from build123d import *

# Parameters (mm, degrees)
F1_DEPTH = 152.4


# Not quite as in the source:
# - ends of sketch curves that miss each other by under 0.0002 mm in the source are joined


with BuildPart() as f1:
    # F0 (on Front) → F1 (new body)
    with BuildSketch(Plane.XZ):
        with BuildLine():
            ThreePointArc((-3.173984, 31.7550292), (-5.034153519, 36.245875681), (-9.525, 38.1060452))
            Line((-9.525, 38.1060452), (-9.525, -38.1060452))
            ThreePointArc((-9.525, -38.1060452), (-5.034153519, -36.245875681), (-3.173984, -31.7550292))
            ThreePointArc((-3.173984, -31.7550292), (1.3873070975, -29.8232975079), (3.1738358164, -25.2031917651))
            ThreePointArc((3.1738358164, -25.2031917651), (6.6091861803, -22.9435143548), (7.940294, -19.0530226))
            ThreePointArc((7.940294, -19.0530226), (7.2093686546, -16.094985199), (5.1848340025, -13.817816657))
            ThreePointArc((5.1848340025, -13.817816657), (9.5132844595, -8.141e-06), (5.1848116567, 13.8177933751))
            ThreePointArc((5.1848116567, 13.8177933751), (7.2093653059, 16.0949788365), (7.940294, 19.0530226))
            ThreePointArc((7.940294, 19.0530226), (6.6091861803, 22.9435143548), (3.1738358164, 25.2031917651))
            ThreePointArc((3.1738358164, 25.2031917651), (1.3873169736, 29.8232821056), (-3.173984, 31.7550292))
        make_face()
    extrude(amount=F1_DEPTH)


solid = f1.part
Could you check a few things on this model? Use its own coordinates, in mm. A direction names the side the tool comes from. Give positions to 0.01 mm unless a question says otherwise; leave off trailing zeros. Write each loop counter-clockwise with the first axis right and the second up, starting at its lowest first coordinate (ties: lowest second). Pieces come first, ordered by that corner, then holes. Notation, with made-up numbers: (-14, 12.5) -> (14, 12.5) arc R26 ccw to (14, 32.5) -> close; hole circle Ø2 at (-34, 13). An arc over 180 degrees is marked (long way). Answer as a JSON object with one key per item and string values.
Q1. Which directions (+Z, -Z, +X, -X, +Y, -Y) give clear straight access to the entire face, cutting with the end or side of a thin tool? Please do faces 4 (the cylindrical face through (7.19, -75.13, 16.06)), 5 (the cylindrical face through (-4.99, -75.13, 36.2)).
Taken from the geometry:
{"face 4": "+X, +Y, -Y", "face 5": "+Z, +X, +Y, -Y"}
Q2. Suppose I cut it at C-C on z = 5. Write out the boundary of the cut face in (x, y) (3 decimals), then the cut area to 3 significant figures.
Taken from the geometry:
{"outline": "(-9.525, -152.4) -> (8.992, -152.4) -> (8.992, 0) -> (-9.525, 0) -> close", "area": "2,820 mm²"}
Q3. Suppose I cut it at B-B on x = -1. Write out the boundary of the cut face in (y, z), then the cut area to 3 significant figures.
Taken from the geometry:
{"outline": "(-152.4, -31.37) -> (0, -31.37) -> (0, 31.37) -> (-152.4, 31.37) -> close", "area": "9,560 mm²"}
Q4. Will these pins go through, and if not, where does the flat tip stop? pin 1 Ø8 at (x, y) = (3, -86) entering from -Z; pin 2 Ø8 at (y, z) = (-43, -12) entering from +X; pin 3 Ø3 at (x, y) = (5, -21) entering from +Z; pin 4 Ø1.5 at (x, z) = (-3.5, 16.5) entering from +Y.
Taken from the geometry:
{"pin 1": "stops at z = -31.37", "pin 2": "stops at x = 8.15", "pin 3": "stops at z = 25.11", "pin 4": "stops at y = 0"}
Q5. We'd pull the mould along Z, two halves only. Please class faces 1 (the cylindrical face through (9.512, -75.133, -0.206)), 2 (the flat face through (-9.525, -75, 1)), 3 (the cylindrical face through (6.645, -75.133, 22.897)): released by +Z, released by -Z, zero draft, split by the parting line, or undercut.
Taken from the geometry:
{"face 1": "undercut", "face 2": "zero draft", "face 3": "released by +Z"}
Q6. Please list where these lines run through material, in increasing order: L1, parallel to Z at x = 6, y = -135; L2, parallel to Z at x = 6.5, y = -46; L3, parallel to X at y = -71.5, z = 8.5 (3 decimals).
Taken from the geometry:
{"L1": "z = -23.62 to -14.48, -12.56 to 12.56, 14.48 to 23.62", "L2": "z = -23.08 to -15.03, -11.7 to 11.7, 15.03 to 23.08", "L3": "x = -9.525 to 7.973"}
Q7. Suppose I cut it at A-A on y = -64.5. Write out the boundary of the cut face in (x, z) (3 decimals).
Taken from the geometry:
{"outline": "(-9.525, -38.106) arc R6.351 ccw to (-3.174, -31.755) arc R6.351 ccw to (3.174, -25.203) arc R6.351 ccw to (5.185, -13.818) arc R24.22 ccw to (5.185, 13.818) arc R6.351 ccw to (7.94, 19.053) arc R6.351 ccw to (3.174, 25.203) arc R6.351 ccw to (-3.174, 31.755) arc R6.351 ccw to (-9.525, 38.106) -> close"}
